```python
from build123d import *

# Parameters (mm, degrees)
AUFSATZ_LINEAR_AUSTRAGEN1_DEPTH      = 80
AUFSATZ_LINEAR_AUSTRAGEN1_DEPTH_BACK = 15
SKIZZE1_W                            = 207
SKIZZE1_H                            = 32
SKIZZE1_R                            = 9.5
SKIZZE2_R                            = 12.5
SCHNITT_LINEAR_AUSTRAGEN1_DEPTH      = 31
SCHNITT_LINEAR_START                 = -31
SKIZZE3_R                            = 12.5
SCHNITT_LINEAR_AUSTRAGEN2_DEPTH      = 31
SCHNITT_LINEAR_AUSTRAGEN3_DEPTH      = 132.788656568
SCHNITT_LINEAR_AUSTRAGEN3_DEPTH_BACK = 5
SKIZZE4_R                            = 7.5
SKIZZE6_W                            = 143
SKIZZE6_H                            = 55
SCHNITT_LINEAR_AUSTRAGEN5_DEPTH      = 135.670895148
AUFSATZ_LINEAR_AUSTRAGEN2_DEPTH      = 5
AUFSATZ_LINEAR_AUSTRAGEN2_DEPTH_BACK = 1.5
SKIZZE5_R                            = 1.55
SCHNITT_LINEAR_AUSTRAGEN6_DEPTH      = 204.238775828
SCHNITT_LINEAR_AUSTRAGEN6_DEPTH_BACK = 204.238775828
SKIZZE8_W                            = 99.5
SKIZZE8_H                            = 26
SKIZZE8_W_2                          = 39.5
F_2_5_2_5_DURCHMESSER_BOHRUNG2_D     = 2.5
F_2_5_2_5_DURCHMESSER_BOHRUNG2_DEPTH = 10
F_2_5_2_5_DURCHMESSER_BOHRUNG2_TIP   = 1.25
F_2_5_2_5_DURCHMESSER_BOHRUNG1_D     = 2.5
F_2_5_2_5_DURCHMESSER_BOHRUNG1_DEPTH = 10
F_2_5_2_5_DURCHMESSER_BOHRUNG1_TIP   = 1.25
SCHNITT_LINEAR_AUSTRAGEN7_DEPTH      = 2
AUFSATZ_LINEAR_AUSTRAGEN3_DEPTH      = 67.5
SCHNITT_LINEAR_AUSTRAGEN8_DEPTH      = 12
AUFSATZ_LINEAR_AUSTRAGEN4_DEPTH      = 29
SCHNITT_LINEAR_AUSTRAGEN9_DEPTH      = 26
VERRUNDUNG1_R                        = 10
SKIZZE20_W                           = 143
SKIZZE20_H                           = 3
AUFSATZ_LINEAR_AUSTRAGEN5_DEPTH      = 3
SCHNITT_LINEAR_AUSTRAGEN10_DEPTH     = 214.187710715
SCHNITT_LINEAR_AUSTRAGEN11_DEPTH     = 212.378806885
VERRUNDUNG2_R                        = 2.5
SKIZZE23_W                           = 4
SKIZZE23_H                           = 2
AUFSATZ_LINEAR_AUSTRAGEN6_DEPTH      = 2


with BuildPart() as part:
    # Skizze1 → Aufsatz-Linear austragen1 (new, two sides: drawn at the far end of the back side and taken through both)
    with BuildSketch(Plane(origin=(0, 0, 0), x_dir=(1, 0, 0), z_dir=(0, 1, 0)).offset(-AUFSATZ_LINEAR_AUSTRAGEN1_DEPTH_BACK)):
        Rectangle(SKIZZE1_W, SKIZZE1_H)
        with Locations(Location((-87.5, 0, 0), (0, 0, 270))):
            Circle(SKIZZE1_R, mode=Mode.SUBTRACT)
        with Locations(Location((87.5, 0, 0), (0, 0, 90))):
            Circle(SKIZZE1_R, mode=Mode.SUBTRACT)
    extrude(amount=AUFSATZ_LINEAR_AUSTRAGEN1_DEPTH + AUFSATZ_LINEAR_AUSTRAGEN1_DEPTH_BACK)

    # Skizze2 → Schnitt-Linear austragen1 (cut)
    with BuildSketch(Plane(origin=(0, 80, 0), x_dir=(1, 0, 0), z_dir=(0, 1, 0))):
        with Locations(Location((-87.5, 0, 0), (0, 0, 270))):
            Circle(SKIZZE2_R)
        with Locations(Location((87.5, 0, 0), (0, 0, 270))):
            Circle(SKIZZE2_R)
    extrude(amount=-SCHNITT_LINEAR_AUSTRAGEN1_DEPTH, mode=Mode.SUBTRACT)

    # Skizze3 → Schnitt-Linear austragen2 (cut)
    with BuildSketch(Plane.XZ.offset(15).offset(SCHNITT_LINEAR_START)):
        with Locations(Location((-87.5, 0, 0), (0, 0, 90))):
            Circle(SKIZZE3_R)
        with Locations(Location((87.5, 0, 0), (0, 0, 90))):
            Circle(SKIZZE3_R)
    extrude(amount=SCHNITT_LINEAR_AUSTRAGEN2_DEPTH, mode=Mode.SUBTRACT)

    # Skizze4 → Schnitt-Linear austragen3 (cut, two sides: drawn at the far end of the back side and taken through both)
    with BuildSketch(Plane.XY.offset(-SCHNITT_LINEAR_AUSTRAGEN3_DEPTH_BACK)):
        with Locations((-20, 0)):
            Circle(SKIZZE4_R)
        Polygon((-38.414213562, 10), (-37, 11.414213562), (-35.585786438, 10), (-37, 8.585786438), align=None)
        Polygon((-35.585786438, -10), (-37, -8.585786438), (-38.414213562, -10), (-37, -11.414213562), align=None)
    extrude(amount=SCHNITT_LINEAR_AUSTRAGEN3_DEPTH + SCHNITT_LINEAR_AUSTRAGEN3_DEPTH_BACK, mode=Mode.SUBTRACT)

    # Skizze6 → Schnitt-Linear austragen5 (cut, through all)
    with BuildSketch(Plane.XY.offset(16)):
        with Locations((0, 52.5)):
            Rectangle(SKIZZE6_W, SKIZZE6_H)
    extrude(amount=-SCHNITT_LINEAR_AUSTRAGEN5_DEPTH, mode=Mode.SUBTRACT)

    # Skizze5 → Aufsatz-Linear austragen2 (add, two sides: drawn at the far end of the back side and taken through both)
    with BuildSketch(Plane(origin=(0, 0, 0), x_dir=(-1, 0, 0), z_dir=(0, 0, -1)).offset(-AUFSATZ_LINEAR_AUSTRAGEN2_DEPTH_BACK)):
        with BuildLine():
            Line((180, 15), (103.5, 15))
            Line((103.5, 15), (103.5, -15))
            Line((103.5, -15), (180, -15))
            ThreePointArc((180, -15), (195, 0), (180, 15))
        make_face()
        with Locations((180, 8)):
            Circle(SKIZZE5_R, mode=Mode.SUBTRACT)
        with Locations(Location((180, -8, 0), (0, 0, 180))):
            Circle(SKIZZE5_R, mode=Mode.SUBTRACT)
        with BuildLine():
            Line((171, -4), (171, 4))
            ThreePointArc((171, 4), (171.292893219, 4.707106781), (172, 5))
            Line((172, 5), (188, 5))
            ThreePointArc((188, 5), (188.707106781, 4.707106781), (189, 4))
            Line((189, 4), (189, -4))
            ThreePointArc((189, -4), (188.707106781, -4.707106781), (188, -5))
            Line((188, -5), (172, -5))
            ThreePointArc((172, -5), (171.292893219, -4.707106781), (171, -4))
        make_face(mode=Mode.SUBTRACT)
    extrude(amount=AUFSATZ_LINEAR_AUSTRAGEN2_DEPTH + AUFSATZ_LINEAR_AUSTRAGEN2_DEPTH_BACK)

    # Skizze8 → Schnitt-Linear austragen6 (cut, two sides: drawn at the far end of the back side and taken through both)
    with BuildSketch(Plane(origin=(0, 25, 0), x_dir=(1, 0, 0), z_dir=(0, 1, 0)).offset(-SCHNITT_LINEAR_AUSTRAGEN6_DEPTH_BACK)):
        with Locations((-21.75, 0)):
            Rectangle(SKIZZE8_W, SKIZZE8_H)
        with Locations((51.75, 0)):
            Rectangle(SKIZZE8_W_2, SKIZZE8_H)
    extrude(amount=SCHNITT_LINEAR_AUSTRAGEN6_DEPTH + SCHNITT_LINEAR_AUSTRAGEN6_DEPTH_BACK, mode=Mode.SUBTRACT)

    # Ø2.5 (2.5) Durchmesser Bohrung2
    with Locations(Plane(origin=(0, 80, 0), x_dir=(1, 0, 0), z_dir=(0, 1, 0))):
        with Locations((75.511004525, -11.988995475), (99.488995475, -11.988995475), (75.511004525, 11.988995475), (99.488995475, 11.988995475), (-75.511004525, 11.988995475), (-99.488995475, 11.988995475), (-75.511004525, -11.988995475), (-99.488995475, -11.988995475)):
            Hole(F_2_5_2_5_DURCHMESSER_BOHRUNG2_D / 2, depth=F_2_5_2_5_DURCHMESSER_BOHRUNG2_DEPTH)
            with Locations((0, 0, -(F_2_5_2_5_DURCHMESSER_BOHRUNG2_DEPTH + F_2_5_2_5_DURCHMESSER_BOHRUNG2_TIP / 2))):  # 90° drill point
                Cone(0, F_2_5_2_5_DURCHMESSER_BOHRUNG2_D / 2, F_2_5_2_5_DURCHMESSER_BOHRUNG2_TIP, mode=Mode.SUBTRACT)

    # Ø2.5 (2.5) Durchmesser Bohrung1
    with Locations(Plane(origin=(0, -15, 0), x_dir=(-1, 0, 0), z_dir=(0, -1, 0))):
        with Locations((-75.511004525, 11.988995475), (-99.488995475, 11.988995475), (-99.488995475, -11.988995475), (-75.511004525, -11.988995475), (75.511004525, 11.988995475), (99.488995475, 11.988995475), (75.511004525, -11.988995475), (99.488995475, -11.988995475)):
            Hole(F_2_5_2_5_DURCHMESSER_BOHRUNG1_D / 2, depth=F_2_5_2_5_DURCHMESSER_BOHRUNG1_DEPTH)
            with Locations((0, 0, -(F_2_5_2_5_DURCHMESSER_BOHRUNG1_DEPTH + F_2_5_2_5_DURCHMESSER_BOHRUNG1_TIP / 2))):  # 90° drill point
                Cone(0, F_2_5_2_5_DURCHMESSER_BOHRUNG1_D / 2, F_2_5_2_5_DURCHMESSER_BOHRUNG1_TIP, mode=Mode.SUBTRACT)

    # Skizze13 → Schnitt-Linear austragen7 (cut)
    with BuildSketch(Plane.XY.offset(1.5)):
        with BuildLine():
            Line((-180, 15), (-103.5, 15))
            Line((-103.5, 15), (-103.5, -15))
            Line((-103.5, -15), (-180, -15))
            ThreePointArc((-180, -15), (-165, 0), (-180, 15))
        make_face()
    extrude(amount=-SCHNITT_LINEAR_AUSTRAGEN7_DEPTH, mode=Mode.SUBTRACT)

    # Skizze14 → Aufsatz-Linear austragen3 (add)
    with BuildSketch(Plane.ZY.offset(103.5)):
        Polygon((-5, -15), (-13.5, -15), (-13.5, -7.221825407), (-5, 1.278174593), (-5, 1.222837222), align=None)
        with BuildLine():
            Line((-10.621320344, -7.878679656), (-8.5, -5.757359313))
            Line((-8.5, -5.757359313), (-6.378679656, -7.878679656))
            ThreePointArc((-6.378679656, -7.878679656), (-8.5, -13), (-10.621320344, -7.878679656))
        make_face(mode=Mode.SUBTRACT)
    extrude(amount=AUFSATZ_LINEAR_AUSTRAGEN3_DEPTH)

    # Skizze15 → Schnitt-Linear austragen8 (cut)
    with BuildSketch(Plane.XY.offset(16)):
        Polygon((66.75, 20.5), (68, 21.75), (69.25, 20.5), (68, 19.25), align=None)
        Polygon((68, -8.75), (69.25, -10), (68, -11.25), (66.75, -10), align=None)
    extrude(amount=-SCHNITT_LINEAR_AUSTRAGEN8_DEPTH, mode=Mode.SUBTRACT)

    # Skizze17 → Aufsatz-Linear austragen4 (add)
    with BuildSketch(Plane(origin=(0, 0, -16), x_dir=(-1, 0, 0), z_dir=(0, 0, -1))):
        Polygon((39, 25), (35, 25), (35, 15.071067812), (29.928932188, 10), (35, 4.928932188), (35, -4.928932188), (29.928932188, -10), (35, -15.071067812), (35, -15), (39, -15), (39, -15.071067812), (44.071067812, -10), (39, -4.928932188), (39, 4.928932188), (44.071067812, 10), (39, 15.071067812), align=None)
        Polygon((37, 11.414213562), (35.585786438, 10), (37, 8.585786438), (38.414213562, 10), align=None, mode=Mode.SUBTRACT)
        Polygon((37, -8.585786438), (38.414213562, -10), (37, -11.414213562), (35.585786438, -10), align=None, mode=Mode.SUBTRACT)
    extrude(amount=-AUFSATZ_LINEAR_AUSTRAGEN4_DEPTH)

    # Skizze18 → Schnitt-Linear austragen9 (cut)
    with BuildSketch(Plane(origin=(0, 0, -16), x_dir=(-1, 0, 0), z_dir=(0, 0, -1))):
        Polygon((32.898780669, 10), (37, 14.101219331), (41.101219331, 10), (37, 5.898780669), align=None)
        Polygon((32.898780669, -10), (37, -5.898780669), (41.101219331, -10), (37, -14.101219331), align=None)
    extrude(amount=-SCHNITT_LINEAR_AUSTRAGEN9_DEPTH, mode=Mode.SUBTRACT)

    # Verrundung1
    verrundung1_edges = [part.edges().sort_by_distance(p)[0] for p in [
        (-103.5, 15, -2.75),
        (-103.5, 0, -0.5),
    ]]
    fillet(verrundung1_edges, radius=VERRUNDUNG1_R)

    # Skizze20 → Aufsatz-Linear austragen5 (add)
    with BuildSketch(Plane(origin=(0, 25, 0), x_dir=(1, 0, 0), z_dir=(0, 1, 0))):
        with Locations((0, 14.5)):
            Rectangle(SKIZZE20_W, SKIZZE20_H)
    extrude(amount=AUFSATZ_LINEAR_AUSTRAGEN5_DEPTH)

    # Skizze21 → Schnitt-Linear austragen10 (cut, through all)
    with BuildSketch(Plane.XY.offset(16)):
        Polygon((0, 22.414213562), (-1.414213562, 21), (0, 19.585786438), (1.414213562, 21), align=None)
    extrude(amount=-SCHNITT_LINEAR_AUSTRAGEN10_DEPTH, mode=Mode.SUBTRACT)

    # Skizze22 → Schnitt-Linear austragen11 (cut, through all)
    with BuildSketch(Plane.XY):
        Polygon((-87.5, 41.25), (-88.75, 40), (-87.5, 38.75), (-86.25, 40), align=None)
        Polygon((87.5, 41.25), (86.25, 40), (87.5, 38.75), (88.75, 40), align=None)
    extrude(amount=SCHNITT_LINEAR_AUSTRAGEN11_DEPTH, mode=Mode.SUBTRACT)

    # Verrundung2
    verrundung2_edges = [part.edges().sort_by_distance(p)[0] for p in [
        (-37, 5.898780669, -3),
        (-37, -14.101219331, -3),
    ]]
    fillet(verrundung2_edges, radius=VERRUNDUNG2_R)

    # Skizze23 → Aufsatz-Linear austragen6 (add)
    with BuildSketch(Plane(origin=(0, 25, 0), x_dir=(1, 0, 0), z_dir=(0, 1, 0))):
        with Locations((-37, -6)):
            Rectangle(SKIZZE23_W, SKIZZE23_H)
        with Locations((30, -6)):
            Rectangle(SKIZZE23_W, SKIZZE23_H)
    extrude(amount=AUFSATZ_LINEAR_AUSTRAGEN6_DEPTH)


solid = part.part
```
Part model, mm, in its own coordinate system. A direction names the side the tool comes from. Round coordinates to 2 decimals unless told otherwise and drop trailing zeros. Order: outer loops, then holes, each group sorted by start corner. A loop starts at its lowest first (then second) coordinate and runs counter-clockwise, first axis right, second up. Notation, with made-up numbers: M 34,-2 L 53,-2 A19 ccw 53,30 Z; hole C 44,30.5 d8. An arc over 180 degrees is marked long. Put each result on its own line as item: value. Start each with the question number.
1. Tool access for faces 4 (the face through (-136.8, -13, -8.4)), 5 (the face through (-149, 5, -5)), 6 (the face through (-41.5, -12.57, -1.7)): list every direction of +Z, -Z, +X, -X, +Y, -Y with a clear straight run to the whole face (end or side of a thin tool).
2. Drill centre lines: probe 1 along Z at (x, y) = (87, 52.5); probe 2 along X at (y, z) = (73, 2); probe 3 along X at (y, z) = (-9.5, 14). Where is each one in solid material? Low to high. Write a range as [from, to].
3. Slice it at C-C on x = -59.5. List the corners of the cut face in (y, z), then the cut area to 3 significant figures.
4. Slice it at A-A on y = 56.5. List the corners of the cut face in (x, z).
5. Slice it at D-D on x = 82. List the corners of the cut face in (y, z).
6. Drop flat-ended pins along their axis: pin 1 (3.5 mm diameter, centred on x = -180, y = -8, fed in from -Z); pin 2 (5 mm diameter, centred on x = -42.5, z = 0.5, fed in from -Y); pin 3 (2 mm diameter, centred on x = 99.49, z = 11.99, fed in from +Y). Give the stop position or say it passes through.
7. Two-plate mould, pull along X, no slides. Class faces 1 (the face through (99.894, 64.717, -1.627)), 2 (the face through (-180, -6, 1.5)), 3 (the face through (-103.5, 42, 0)): +X half, -X half, draft (parallel to the pull), parting line (faces both ways), or undercut.
8. Slice it at B-B on x = -20. List the corners of the cut face in (y, z), then the cut area to 3 significant figures.
Findings:
1. face 4: -X
1. face 5: -Z, -X, +Y
1. face 6: -Y
2. probe 1: [-16, -12.49], [12.49, 16]
2. probe 2: [-103.5, -99.84], [-75.16, -71.5], [71.5, 75.16], [99.84, 103.5]
2. probe 3: [-103.5, -37.91], [-36.09, 67.25], [68.75, 103.5]
3. outline: M -15,-16 L 28,-16 L 28,-13 L -15,-13 Z; M -15,13 L 25,13 L 25,16 L -15,16 Z
3. area: 249 mm2
4. outline: M -103.5,-16 L -71.5,-16 L -71.5,16 L -103.5,16 Z; M 71.5,-16 L 103.5,-16 L 103.5,16 L 71.5,16 Z; hole C -87.5,0 d25; hole C 87.5,0 d25
5. outline: M -15,-16 L 80,-16 L 80,-11.22 L 49,-11.22 L 49,-7.75 L 16,-7.75 L 16,-11.22 L -15,-11.22 Z; M -15,11.22 L 16,11.22 L 16,7.75 L 49,7.75 L 49,11.22 L 80,11.22 L 80,16 L -15,16 Z
6. pin 1: z = -5
6. pin 2: y = -14.07
6. pin 3: y = 69.75
7. face 1: undercut
7. face 2: draft
7. face 3: -X half
8. outline: M -15,-16 L 28,-16 L 28,-13 L -15,-13 Z; M -15,13 L -7.5,13 L -7.5,16 L -15,16 Z; M 7.5,13 L 25,13 L 25,16 L 7.5,16 Z
8. area: 204 mm2
